Drawing for the job (mm, zero at the part's lowest x, y, z). Coordinates: 2 decimals unless noted, no trailing zeros. Loops run counter-clockwise (first coordinate to the right, second up) from the corner with the lowest first, then second, coordinate; pieces in that order, holes last. Notation, with made-up numbers: (71, -5.5) -> (128, -5.5) arc R13 ccw to (128, 19.5) -> close; hole circle Ø6 at (43, 13). An arc over 180 degrees is marked (long way). Write each question's results on one line, items separated by ' | '.
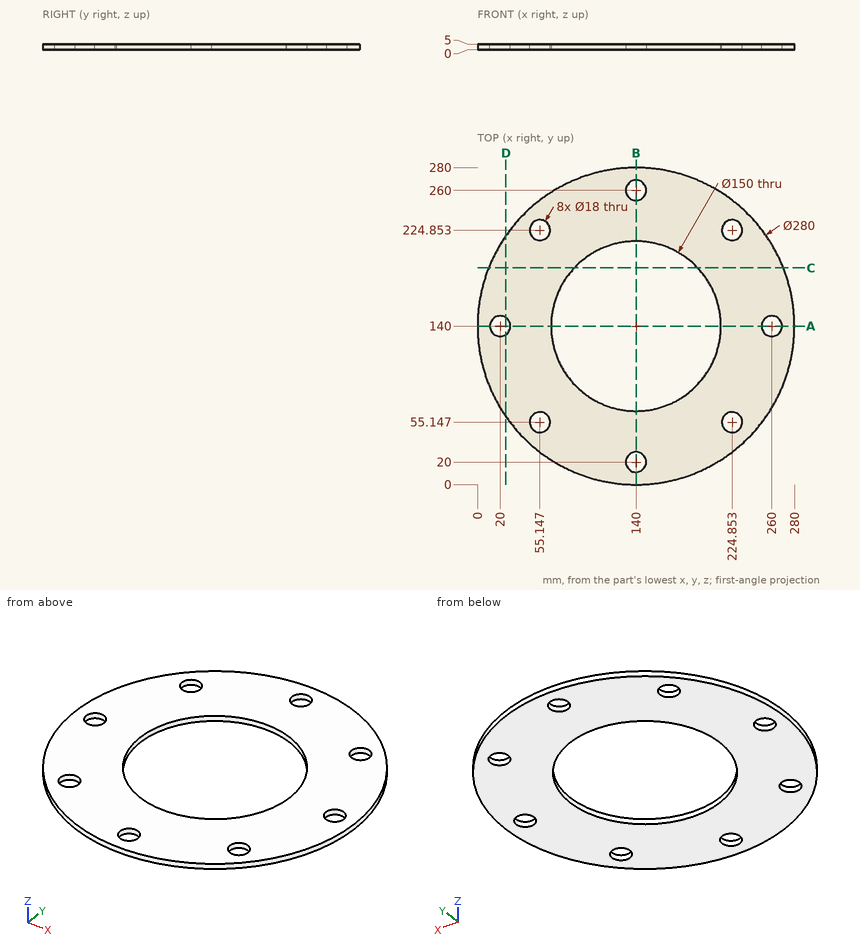
1) Slice it at C-C (y = 191.5). Write the cut outline in (x, z).
Outcome:
outline: (9.82, 0) -> (85.48, 0) -> (85.48, 5) -> (9.82, 5) -> close; (194.52, 0) -> (270.18, 0) -> (270.18, 5) -> (194.52, 5) -> close
2) Drill centre lines: L1, parallel to Y at x = 140, z = 2.95; L2, parallel to Y at x = 60, z = 2.5; L3, parallel to Y at x = 223, z = 3.8 (1 decimal). Where is each one in solid material? Low to high. Write a range as from..to.
Outcome:
L1: y = 0..11, 29..65, 215..251, 269..280 | L2: y = 25.11..47.57, 62.73..217.27, 232.43..254.89 | L3: y = 27.3..46.3, 64..216, 233.7..252.7
3) Slice it at A-A (y = 140). Write the cut outline in (x, z), then the cut area to 3 significant figures.
Outcome:
outline: (0, 0) -> (11, 0) -> (11, 5) -> (0, 5) -> close; (29, 0) -> (65, 0) -> (65, 5) -> (29, 5) -> close; (215, 0) -> (251, 0) -> (251, 5) -> (215, 5) -> close; (269, 0) -> (280, 0) -> (280, 5) -> (269, 5) -> close | area: 470 mm^2
4) Pin check, flat tip, straight feed: pin 1 (23.5 mm diameter, centred on x = 55.15, y = 224.85, fed in from -Z). Stop position of the tip, or through.
Outcome:
pin 1: stops at z = 0
5) Slice it at D-D (x = 25). Write the cut outline in (y, z).
Outcome:
outline: (60.16, 0) -> (132.52, 0) -> (132.52, 5) -> (60.16, 5) -> close; (147.48, 0) -> (219.84, 0) -> (219.84, 5) -> (147.48, 5) -> close
